Source: three-view drawing plus pictorial views. Frame: mm from the lowest corner of the part. Give positions to 0.01 mm unless a question says otherwise; leave off trailing zeros. Order: outer loops, then holes, each group sorted by start corner. A loop starts at its lowest first (then second) coordinate and runs counter-clockwise, first axis right, second up. Notation, with made-up numbers: (32, 39) - (39, 39) arc R13 ccw to (39, 52) - close; hole circle Ø7 at (35.25, 42.5). An arc over 180 degrees is marked (long way). Use CSV: the item, a comma, the result in double quotes.
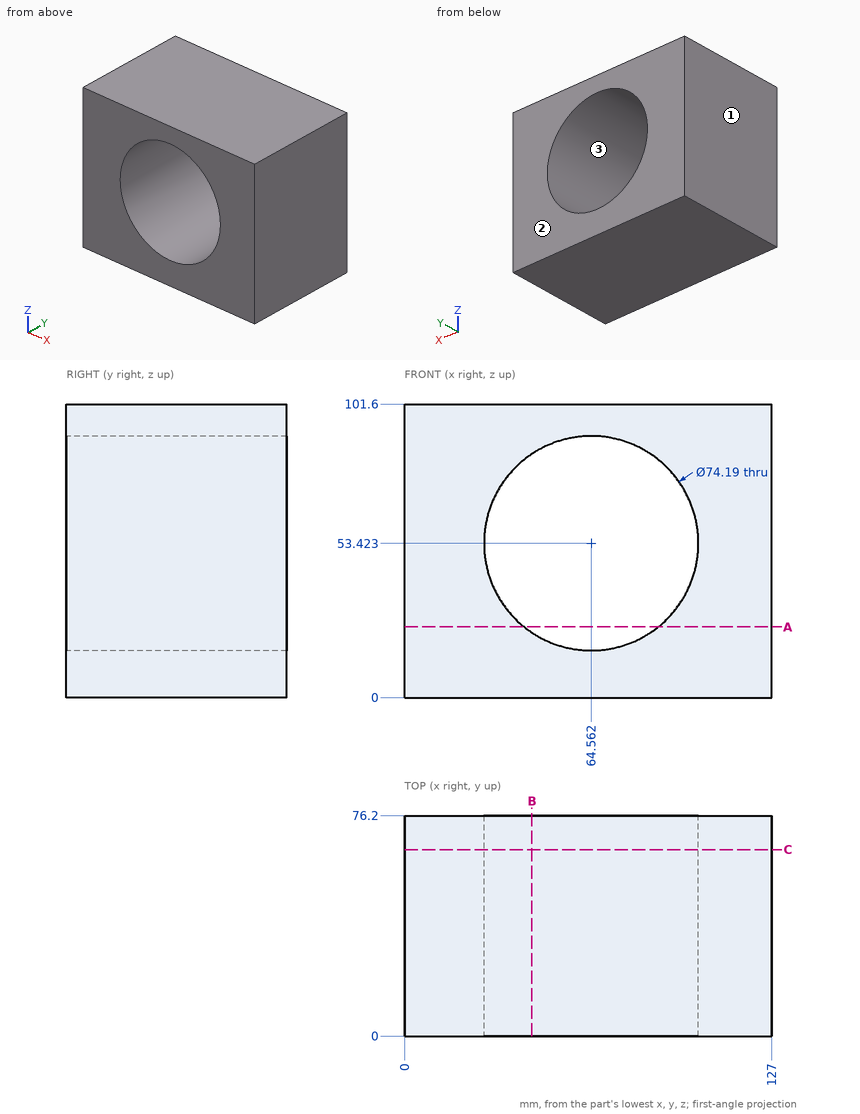
Item 1: Section C-C on y = 64.5. Return the cut outline in (x, z) (1 decimal).
Filled in:
outline,"(0, 0) - (127, 0) - (127, 101.6) - (0, 101.6) - close; hole circle Ø74.2 at (64.6, 53.4)"
Item 2: First-contact query: pin 1 (12 mm diameter, centred on y = 42, z = 32, fed in from -X). Flat tip, straight axial feed; report the tip coordinate or a pass-through.
Filled in:
pin 1,"stops at x = 0"
Item 3: Mould query, pull axis X, two halves, no side actions, for the marked faces 1, 2 and 3. Classes: released by +X, released by -X, zero draft, split by the parting line, or undercut.
Filled in:
face 1,"released by -X"
face 2,"zero draft"
face 3,"undercut"
Item 4: Section A-A on z = 24.5. Return the cut outline in (x, y) (1 decimal), then the cut area to 3 significant figures.
Filled in:
outline,"(0, 0) - (41.3, 0) - (41.3, 76.2) - (0, 76.2) - close; (87.8, 0) - (127, 0) - (127, 76.2) - (87.8, 76.2) - close"
area,"6,140 mm2"
Item 5: Section B-B on x = 44. Return the cut outline in (y, z).
Filled in:
outline,"(0, 0) - (76.2, 0) - (76.2, 22.55) - (0, 22.55) - close; (0, 84.3) - (76.2, 84.3) - (76.2, 101.6) - (0, 101.6) - close"
Item 6: Material intervals for line 1 (X direction, y = 24.5, z = 77) (1 decimal); line 2 (X direction, y = 18, z = 73.5) (1 decimal); line 3 (Z direction, x = 60, y = 60) (1 decimal), sorted ascending. Write a range as from..to.
Filled in:
line 1,"x = 0..35.9, 93.2..127"
line 2,"x = 0..33.4, 95.8..127"
line 3,"z = 0..16.6, 90.2..101.6"
